Source: CAD feature listing. Evaluate the final solid. Frame: model axes, mm. A direction names the side the tool comes from. Coordinates: 2 decimals unless noted, no trailing zeros. Order: outer loops, then holes, each group sorted by start corner. A loop starts at its lowest first (then second) coordinate and runs counter-clockwise, first axis right, second up. Notation, with made-up numbers: (35.5, 38.25) -> (57.5, 38.25) arc R16 ccw to (57.5, 69.25) -> close; hole circle Ø3 at (29.25, -5). An arc over 180 degrees is marked (long way). Write item = value, one per line. Start each with the question number.
Item 1: Set-up query: faces 4 (the cylindrical face through (-0.09, 4.3, -7.05)), 5 (the cylindrical face through (-0.07, 4.55, 3.45)). Return all of +Z, -Z, +X, -X, +Y, -Y with unobstructed straight access to the full face (end or side cutting, diameter ignored); none if empty.
Item 2: Ray query, line 1 along X through (y, z) = (0.1, 0); line 2 along X through (y, z) = (1.25, -5); line 3 along Z through (x, y) = (-1, 7.75). Return the intervals inside material, ascending. Write a range as [from, to].
Item 3: Mould query, pull axis X, two halves, no side actions, for faces 1 (the cylindrical face through (-1.952, 7.754, -0.434)), 2 (the cylindrical face through (13.856, 0.26, 5.745)), 3 (the flat face through (2, 8, 2)). Classes: released by +X, released by -X, zero draft, split by the parting line, or undercut.
Item 4: Section query B-B (x = 0). Count the separate pieces of the cut face and the enclosed holes in it, then the cut area to 3 significant figures.
Item 5: Section query A-A (y = 6). Output: boundary loops of the cut face in (x, z), then the cut area to 3 significant figures.
Item 6: Contact query for flat-ended pins moving along their axis: pin 1 (1 mm diameter, centred on y = 7, z = -10, fed in from +X); pin 2 (3 mm diameter, centred on x = -10.5, y = 1, fed in from +Z); pin 3 (2 mm diameter, centred on x = -1, z = -5.5, fed in from -Y); pin 4 (1 mm diameter, centred on y = 1.5, z = -4.5, fed in from -X). Output: stop coordinate, or through.
```python
from build123d import *

# Parameters (mm, degrees)
CROQUIS5_R              = 2
CORTAR_EXTRUIR1_DEPTH   = 6
CROQUIS6_R              = 14.5
CORTAR_EXTRUIR2_DEPTH   = 0.5
CROQUIS7_R              = 2.05
CROQUIS7_R_2            = 1.55
SALIENTE_EXTRUIR1_DEPTH = 6.5
CORTAR_EXTRUIR3_START   = -5.5
CROQUIS8_R              = 1.55
CORTAR_EXTRUIR3_DEPTH   = 5.5
REDONDEO1_R             = 2
REDONDEO2_R             = 2


with BuildPart() as part:
    # Croquis3 → Revolución1 (revolve)
    with BuildSketch(Plane.XY):
        with BuildLine():
            Line((15, 0), (15, 1.694213924))
            ThreePointArc((15, 1.694213924), (12.549846274, 2.962329925), (9.993557502, 4))
            ThreePointArc((9.993557502, 4), (9.70509179, 6.051742746), (9, 8))
            Line((9, 8), (0, 8))
            Line((0, 8), (0, 0))
            Line((0, 0), (15, 0))
        make_face()
    revolve(axis=Axis((0, 0, 0), (0, 1, 0)))

    # Croquis4 → Cortar-Revolución1 (revolve, cut)
    with BuildSketch(Plane.XY):
        with BuildLine():
            Line((0, 0.5), (0, 7.5))
            Line((0, 7.5), (8.680950348, 7.5))
            ThreePointArc((8.680950348, 7.5), (9.292895722, 5.613938885), (9.499999964, 3.641931911))
            ThreePointArc((9.499999964, 3.641931911), (12.052061122, 2.639235415), (14.5, 1.403916968))
            Line((14.5, 1.403916968), (14.5, 0.5))
            Line((14.5, 0.5), (0, 0.5))
        make_face()
    revolve(axis=Axis((0, 7.5, 0), (0, 1, 0)), mode=Mode.SUBTRACT)

    # Croquis5 → Cortar-Extruir1 (cut)
    with BuildSketch(Plane(origin=(0, 8, 0), x_dir=(1, 0, 0), z_dir=(0, 1, 0))):
        with Locations(Location((0, 0, 0), (0, 0, 270))):
            Circle(CROQUIS5_R)
    extrude(amount=-CORTAR_EXTRUIR1_DEPTH, mode=Mode.SUBTRACT)

    # Croquis6 → Cortar-Extruir2 (cut)
    with BuildSketch(Plane.XZ):
        Circle(CROQUIS6_R)
    extrude(amount=-CORTAR_EXTRUIR2_DEPTH, mode=Mode.SUBTRACT)

    # Croquis7 → Saliente-Extruir1 (add)
    # profile 1 of 2: a face of its own
    with BuildSketch(Plane.XZ.offset(-7.5)):
        with Locations(Location((0, 5, 0), (0, 0, 90))):
            Circle(CROQUIS7_R)
        with Locations(Location((0, 5, 0), (0, 0, 90))):
            Circle(CROQUIS7_R_2, mode=Mode.SUBTRACT)
    # profile 2 of 2: a face of its own
    with BuildSketch(Plane.XZ.offset(-7.5)):
        with Locations(Location((0, -5, 0), (0, 0, 90))):
            Circle(CROQUIS7_R)
        with Locations(Location((0, -5, 0), (0, 0, 90))):
            Circle(CROQUIS7_R_2, mode=Mode.SUBTRACT)
    extrude(amount=SALIENTE_EXTRUIR1_DEPTH)

    # Croquis8 → Cortar-Extruir3 (cut)
    with BuildSketch(Plane.XZ.offset(-7.5).offset(CORTAR_EXTRUIR3_START)):
        with Locations(Location((0, -5, 0), (0, 0, 90))):
            Circle(CROQUIS8_R)
        with Locations(Location((0, 5, 0), (0, 0, 90))):
            Circle(CROQUIS8_R)
    extrude(amount=CORTAR_EXTRUIR3_DEPTH, mode=Mode.SUBTRACT)

    # Redondeo1
    redondeo1_edges = [part.edges().sort_by_distance(p)[0] for p in [
        (-9, 8, 0),
    ]]
    fillet(redondeo1_edges, radius=REDONDEO1_R)

    # Redondeo2
    redondeo2_edges = [part.edges().sort_by_distance(p)[0] for p in [
        (-15, 1.694213924, 0),
    ]]
    fillet(redondeo2_edges, radius=REDONDEO2_R)


solid = part.part
```
Computed:
q1.face_4 = -Y
q1.face_5 = +Y, -Y
q2.line_1 = [-15, -14.5], [14.5, 15]
q2.line_2 = [-13.99, -13.61], [-2.05, -1.55], [1.55, 2.05], [13.61, 13.99]
q2.line_3 = [-8.55, -6.18], [-3.82, -1.73], [1.73, 3.82], [6.18, 8.55]
q3.face_1 = undercut
q3.face_2 = split by the parting line
q3.face_3 = zero draft
q4.separate_pieces = 4
q4.enclosed_holes = 0
q4.area = 26.7 mm^2
q5.outline = circle Ø19.44 at (0, 0); circle Ø4.1 at (0, -5); circle Ø4.1 at (0, 5); hole circle Ø18.4 at (0, 0); hole circle Ø3.1 at (0, -5); hole circle Ø3.1 at (0, 5)
q5.area = 41.9 mm^2
q6.pin_1 = through
q6.pin_2 = 11.97
q6.pin_3 = 1
q6.pin_4 = -14.31
